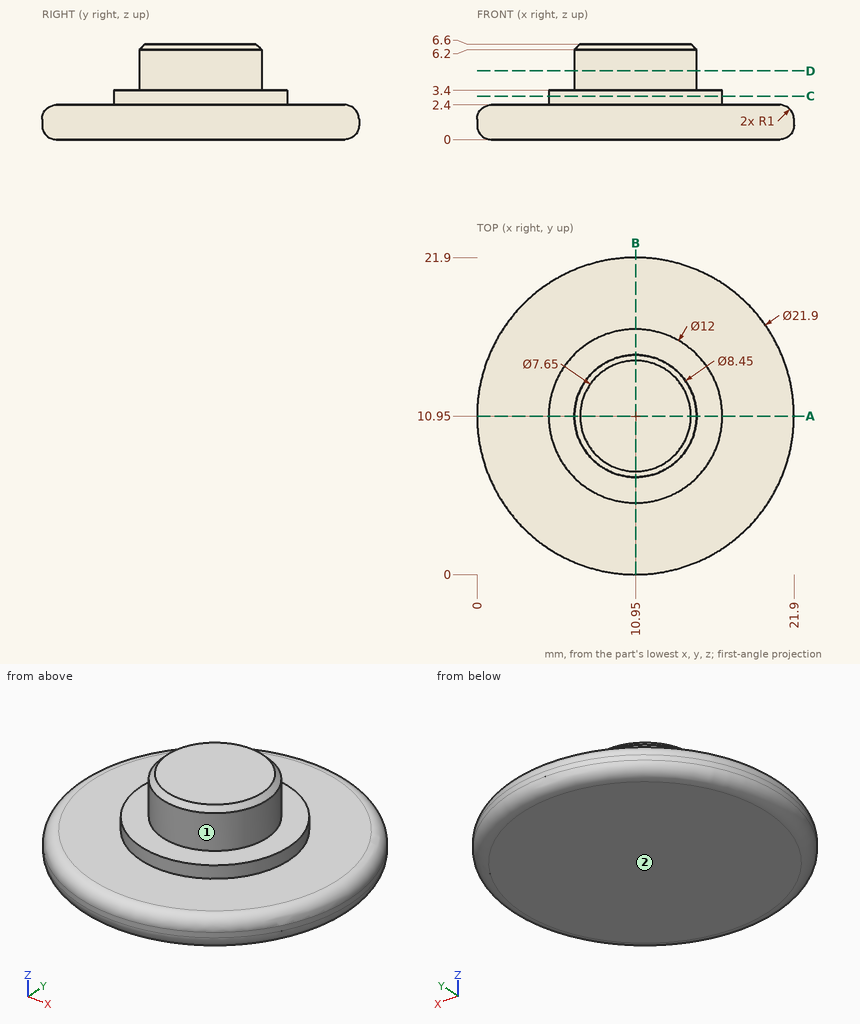
For this review, use the dimensioned drawing (mm, ordinates from the lowest corner) and the shaded views. A direction names the side the tool comes from. Give positions to 0.01 mm unless a question says otherwise; leave off trailing zeros. Loops run counter-clockwise (first coordinate to the right, second up) from the corner with the lowest first, then second, coordinate; pieces in that order, holes last. Notation, with made-up numbers: (-18, 72.5) - (6, 72.5) arc R12 cw to (6, 82.5) - close; hole circle Ø9 at (-36, 36). An arc over 180 degrees is marked (long way). Write each question's results on one line, items separated by ' | '.
(1) Take a section at A-A (y = 10.95). Give the boundary of the cut face in (x, z) (3 decimals).
Conclusion:
outline: (0, 1) arc R1 ccw to (1, 0) - (20.9, 0) arc R1 ccw to (21.9, 1) - (21.9, 1.4) arc R1 ccw to (20.9, 2.4) - (16.95, 2.4) - (16.95, 3.4) - (15.175, 3.4) - (15.175, 6.2) - (14.775, 6.6) - (7.125, 6.6) - (6.725, 6.2) - (6.725, 3.4) - (4.95, 3.4) - (4.95, 2.4) - (1, 2.4) arc R1 ccw to (0, 1.4) - close
(2) For the marked faces 1 and 2, list the 3-axis set-ups (+Z, -Z, +X, -X, +Y, -Y) from which the entire face can be reached by the end or side of a thin tool; tool diameter is ignored.
Conclusion:
face 1: +Z | face 2: -Z, +X, -X, +Y, -Y
(3) Take a section at D-D (z = 4.75). Give the boundary of the cut face in (x, y) (3 decimals).
Conclusion:
outline: circle Ø8.45 at (10.95, 10.95)
(4) Take a section at C-C (z = 3). Give the boundary of the cut face in (x, y).
Conclusion:
outline: circle Ø12 at (10.95, 10.95)
(5) For line 1 along Z through (x, y) = (12.25, 5); line 2 along Z through (x, y) = (15.75, 8.5); line 3 along Y through (x, z) = (9.25, 1), list the stretches that pass through material, from the lowest coordinate up.
Conclusion:
line 1: 0 to 2.4 | line 2: 0 to 3.4 | line 3: 0.13 to 21.77
(6) For pin 1 Ø6 at (x, y) = (15.5, 18) entering from +Z; pin 2 Ø2 at (x, z) = (10.5, 6) entering from -Y (3 decimals); pin 3 Ø1.5 at (x, y) = (12, 19) entering from +Z, all flat-tipped, find the tip position at first contact; note any pin that passes through.
Conclusion:
pin 1: z = 3.4 | pin 2: y = 6.725 | pin 3: z = 2.4
